Here's how the part is built. I have some questions about the finished solid (model axes, mm). Give positions to 0.01 mm unless a question says otherwise; leave off trailing zeros. Order: outer loops, then holes, each group sorted by start corner. A loop starts at its lowest first (then second) coordinate and runs counter-clockwise, first axis right, second up. Notation, with made-up numbers: (-1, 52) -> (33, 52) arc R5 ccw to (33, 61) -> close; hole circle Ø4 at (-12.75, 6). An arc over 180 degrees is marked (long way). Write each question's results on one line, items separated by ' | '. Start each with the question number.
Q1. Imagine slicing it at C-C, the plane z = 1.7. Please give me the cut outline in (x, y) (3 decimals), then the cut area to 3 significant figures.
Q2. Thinking about a two-plate mould opening in X: for faces 1 (the face through (-0.207, 0.133, 0.807)), 2 (the face through (2.381, 0, 2)), 3 (the face through (2, -9.525, 2)), 4 (the face through (-2.381, 0, 2)), which applies, pulls with the +X half, pulls with the -X half, needs draft (parallel to the pull), parting line crosses it, or undercut?
Q3. Imagine slicing it at A-A, the plane x = 0. Please give me the cut outline in (y, z) (1 decimal), then the cut area to 3 significant figures.
Q4. Imagine slicing it at B-B, the plane y = 5.25. Please give me the cut outline in (x, z) (1 decimal).
Q5. I need wall thicknesses on line 1 along X through (y, z) = (-0.25, 2.4); line 2 along Z through (x, y) = (-0.15, 8.25); line 3 along X through (y, z) = (-2.5, 1.65). Which ranges of each line are inside material? Lowest first, please. Write a range as [from, to].
Autodesk Inventor part; units mm, degrees
ref_plane "YZ Plane" through (0, 0, 0) normal (1, 0, 0) x (0, 1, 0)
ref_plane "XZ Plane" through (0, 0, 0) normal (0, 1, 0) x (-1, 0, 0)
ref_plane "XY Plane" through (0, 0, 0) normal (0, 0, 1) x (1, 0, 0)
sketch "Sketch1" plane through (0, 0, 0) normal (0, 0, 1) x (1, 0, 0)
  line L0 (-2.3813, 9.525) -> (2.3813, 9.525)
  line L1 (2.3813, 9.525) -> (2.3813, -9.525)
  line L2 (2.3813, -9.525) -> (-2.3813, -9.525)
  line L3 (-2.3813, -9.525) -> (-2.3813, 9.525)
  point P0 (0, 0)
  point P1 (2.3813, 0)
  point P2 (0, 9.525)
  dimension "d0" = 4.7625
  dimension "d1" = 19.05
extrude "Extrusion1" add sketch "Sketch1" along normal blind 4.7625
sketch "Sketch2" plane through (-2.3813, 9.525, 0) normal (0, 1, 0) x (1, 0, 0)
  circle A0 centre (2.3813, -2.3813) radius 1.5875
  line L0 (0, 0) -> (0, -4.7625)
  line L1 (4.7625, -4.7625) -> (0, -4.7625)
  line L2 (4.7625, 0) -> (0, 0)
  line L3 (4.7625, 0) -> (4.7625, -4.7625)
  point P0 (2.3813, 0)
  dimension "d4" = 3.175
  dimension "d9" = 2.3813
  dimension "d10" = 2.3813
extrude "Extrusion2" cut sketch "Sketch2" against normal through all contours A0
properties part number "ArduinoStilts"
Geometry check:
1) outline: (-2.381, -9.525) -> (-1.434, -9.525) -> (-1.434, 9.525) -> (-2.381, 9.525) -> close; (1.434, -9.525) -> (2.381, -9.525) -> (2.381, 9.525) -> (1.434, 9.525) -> close | area: 36.1 mm²
2) face 1: undercut | face 2: pulls with the +X half | face 3: needs draft | face 4: pulls with the -X half
3) outline: (-9.5, 0) -> (9.5, 0) -> (9.5, 0.8) -> (-9.5, 0.8) -> close; (-9.5, 4) -> (9.5, 4) -> (9.5, 4.8) -> (-9.5, 4.8) -> close | area: 30.2 mm²
4) outline: (-2.4, 0) -> (2.4, 0) -> (2.4, 4.8) -> (-2.4, 4.8) -> close; hole circle Ø3.2 at (0, 2.4)
5) line 1: [-2.38, -1.59], [1.59, 2.38] | line 2: [0, 0.8], [3.96, 4.76] | line 3: [-2.38, -1.41], [1.41, 2.38]
